CAD build for the part. Positions are in the model's coordinates, mm. Coordinates: 2 decimals unless noted, no trailing zeros. Write each loop counter-clockwise with the first axis right and the second up, starting at its lowest first coordinate (ties: lowest second). Pieces come first, ordered by that corner, then holes.
```python
from build123d import *

# Parameters (mm, degrees)
F0_W     = 40
F0_H     = 20
F1_DEPTH = 8
F2_R     = 1.5
F3_DEPTH = 40.001


with BuildPart() as f1:
    # F0 (on Front) → F1 (new body)
    with BuildSketch(Plane.XZ):
        Rectangle(F0_W, F0_H)
    extrude(amount=F1_DEPTH)

    # F2 (on face) → F3 (cut, through all)
    with BuildSketch(Plane(origin=(-20, 0, 0), x_dir=(0, -1, 0), z_dir=(-1, 0, 0))):
        with Locations((4, 4)):
            Circle(F2_R)
        with Locations((4, -4)):
            Circle(F2_R)
    extrude(amount=-F3_DEPTH, mode=Mode.SUBTRACT)


solid = f1.part
```
Item 1: Saw through at A-A, the plane y = -4. Write the cut outline in (x, z).
Item 2: Flat gauge pin, fed straight in: pin 1 Ø2.5 at (y, z) = (-4, -4) entering from +X. Where does the tip first touch, or does it go through?
Item 3: Saw through at C-C, the plane x = 11.5. Write the cut outline in (y, z).
Item 4: Two-plate mould, pull along Z, no slides. Class faces 1 (the cylindrical face through (-0.28, -5.43, 4.45)), 2 (the flat face through (20, -4, 0)), 3 (the flat face through (0, -4, -10)): +Z half, -Z half, draft (parallel to the pull), parting line (faces both ways), or undercut.
Item 5: Wall check: line 1 along Z through (x, y) = (9.5, -4); line 2 along Z through (x, y) = (1.5, -3); line 3 along Y through (x, z) = (-5, -5). Give the ranges that are in metal, low to high.
Item 6: Saw through at B-B, the plane z = 4. Write the cut outline in (x, y).
Working result:
1. outline: (-20, -10) - (20, -10) - (20, -5.5) - (-20, -5.5) - close; (-20, -2.5) - (20, -2.5) - (20, 2.5) - (-20, 2.5) - close; (-20, 5.5) - (20, 5.5) - (20, 10) - (-20, 10) - close
2. pin 1: passes through
3. outline: (-8, -10) - (0, -10) - (0, 10) - (-8, 10) - close; hole circle Ø3 at (-4, -4); hole circle Ø3 at (-4, 4)
4. face 1: undercut
4. face 2: draft
4. face 3: -Z half
5. line 1: z = -10 to -5.5, -2.5 to 2.5, 5.5 to 10
5. line 2: z = -10 to -5.12, -2.88 to 2.88, 5.12 to 10
5. line 3: y = -8 to -5.12, -2.88 to 0
6. outline: (-20, -8) - (20, -8) - (20, -5.5) - (-20, -5.5) - close; (-20, -2.5) - (20, -2.5) - (20, 0) - (-20, 0) - close
